Autodesk Fusion 360 part; units mm, degrees
sketch "Sketch1" plane through (0, 0, 0) normal (0, 0, 1) x (1, 0, 0)
  line L0 (-9, -12) -> (-9, 12)
  line L1 (9, 12) -> (9, -12)
  line L2 (9, -21) -> (-9, 21) construction
  line L3 (-9, -21) -> (9, 21) construction
  line L4 (9, -7.5) -> (-9, -7.5)
  line L5 (-9, -7.5) -> (-9, 7.5)
  line L6 (-9, 7.5) -> (9, 7.5)
  line L7 (9, 7.5) -> (9, -7.5)
  line L8 (9, -7.5) -> (-9, 7.5) construction
  line L9 (-9, -7.5) -> (9, 7.5) construction
  circle A0 centre (0, 0) radius 2.75
  arc A1 (0, 21) -> (-9, 12) centre (0, 12) ccw
  arc A2 (9, 12) -> (0, 21) centre (0, 12) ccw
  arc A3 (0, -21) -> (9, -12) centre (0, -12) ccw
  arc A4 (-9, -12) -> (0, -21) centre (0, -12) ccw
  line L10 (0, -21.9731) -> (0, 33.0269) construction
  line L11 (2.0496, 8.45) -> (4.0992, 12)
  line L12 (4.0992, 12) -> (2.0496, 15.55)
  line L13 (2.0496, 15.55) -> (-2.0496, 15.55)
  line L14 (-2.0496, 15.55) -> (-4.0992, 12)
  line L15 (-4.0992, 12) -> (-2.0496, 8.45)
  line L16 (-2.0496, 8.45) -> (2.0496, 8.45)
  line L17 (2.0496, -15.55) -> (4.0992, -12)
  line L18 (4.0992, -12) -> (2.0496, -8.45)
  line L19 (2.0496, -8.45) -> (-2.0496, -8.45)
  line L20 (-2.0496, -8.45) -> (-4.0992, -12)
  line L21 (-4.0992, -12) -> (-2.0496, -15.55)
  line L22 (-2.0496, -15.55) -> (2.0496, -15.55)
  circle A5 centre (0, 12) radius 2
  circle A6 centre (0, -12) radius 2
  line L23 (-9, 0) -> (0, 0) construction
  line L24 (-3.75, 3.5) -> (-7.25, 3.5)
  line L25 (-7.25, 3.5) -> (-7.25, -3.5)
  line L26 (-7.25, -3.5) -> (-3.75, -3.5)
  line L27 (-3.75, -3.5) -> (-3.75, 3.5)
  line L28 (-3.75, 3.5) -> (-7.25, -3.5) construction
  line L29 (-7.25, 3.5) -> (-3.75, -3.5) construction
  point P0 (0, 12)
  point P1 (0, -12)
  point P2 (-5.5, 0)
  dimension "d14" = 18
  dimension "d15" = 42
  dimension "d16" = 18
  dimension "d17" = 15
  dimension "d18" = 5.5
  dimension "d19" = 9
  dimension "d20" = 12
  dimension "d21" = 12
  dimension "d22" = 3.55
  dimension "d23" = 3.55
  dimension "d24" = 4
  dimension "d25" = 4
  dimension "d26" = 3.5
  dimension "d27" = 7
  dimension "d28" = 3.5
extrude "Extrude1" add sketch "Sketch1" against normal blind 5 contours L0 L1 L4 A3 A4 | L0 L1 L4 L5 L6 L7 | L0 L1 L6 A1 A2 | L11 L12 L13 L14 L15 L16 | L17 L18 L19 L20 L21 L22 | L24 L25 L26 L27
extrude "Extrude2" add sketch "Sketch1" along normal blind 10 contours L0 L1 L4 L5 L6 L7 | L24 L25 L26 L27
extrude "Extrude3" cut sketch "Sketch1" against normal blind 3.5 draft -5 contours L11 L12 L13 L14 L15 L16 | L17 L18 L19 L20 L21 L22 | A5 | A6
extrude "Extrude4" cut sketch "Sketch1" against normal blind 5 from surface at 10 contours L24 L25 L26 L27
sketch "Sketch2" plane through (-3.75, 0, 0) normal (-1, 0, 0) x (0, 0, 1)
  line L0 (10, -3.5) -> (10, 3.5)
  line L1 (10, 3.5) -> (5, 3.5)
  line L2 (5, 3.5) -> (5, -3.5)
  line L3 (5, -3.5) -> (10, -3.5)
  line L4 (9.0415, 0) -> (7.0207, 3.5)
  line L5 (7.0207, 3.5) -> (2.9793, 3.5)
  line L6 (2.9793, 3.5) -> (0.9585, 0)
  line L7 (0.9585, 0) -> (2.9793, -3.5)
  line L8 (2.9793, -3.5) -> (7.0207, -3.5)
  line L9 (7.0207, -3.5) -> (9.0415, 0)
  circle A0 centre (5, 0) radius 2.1
  point P0 (5, 0)
  dimension "d38" = 3.5
  dimension "d41" = 4.2
extrude "Extrude5" cut sketch "Sketch2" along normal up to surface (3.5 mm away) contours L1 L2 L3 L4 L5 L8 L9 A0 | L2 L5 L6 L7 L8 A0 | L2 A0 | L2 A0
extrude "Extrude6" cut sketch "Sketch2" against normal blind 9 from surface at 5.25 contours L2 A0 | L2 A0
chamfer "Chamfer1" distance 0.5 angle 45 19 edges at (-2.5639, 0.9944, 10) (-5.5, 3.5, 10) (-5.5, -3.5, 10) (-7.25, 0, 10) (-9, 0.7594, 3.0421) (-9, 9.75, 0) (0, 21, 0) (9, 9.75, 0) (0, -21, 0) (9, -9.75, 0) (-9, -9.75, 0) (0, 7.5, 10) (9, 0, 10) (0, -7.5, 10) (-9, 0, 10) (-9, 0, -5) (0, 21, -5) (9, 0, -5) (0, -21, -5)
chamfer "Chamfer1" distance 0.5 angle 45 1 edges at (-3.75, 0, 10)
Work out the finished part from the listing and answer in its coordinate system (mm). A direction names the side the tool comes from. Give positions to 0.01 mm unless a question says otherwise; leave off trailing zeros. Order: outer loops, then holes, each group sorted by start corner. A loop starts at its lowest first (then second) coordinate and runs counter-clockwise, first axis right, second up. Notation, with made-up numbers: (82, -14.75) -> (90, -14.75) arc R11 cw to (90, 4.25) -> close; hole circle Ø3 at (34.5, 85.5). An arc over 180 degrees is marked (long way). Answer as a JSON object with one key per item and string values. Group by question number.
1. A tool of negligible diameter and unlimited length cuts with its end or side. For faces 5 (the flat face through (0, 17, 0)), 6 (the cylindrical face through (-7.884, 0.631, 7.003)), 7 (the flat face through (0, -8.6, -1.7)), from which of +Z, -Z, +X, -X, +Y, -Y can it reach the whole face along a straight path? Write none if from no direction.
2. Flat-ended cylindrical pins translate along their axes: pin 1 Ø5 at (y, z) = (0, 5) entering from -X; pin 2 Ø1.9 at (x, y) = (1, 10.5) entering from +Z; pin 3 Ø1 at (x, z) = (-5.5, 6) entering from +Y; pin 4 Ø3.5 at (x, y) = (0, -12) entering from +Z. Find the tip coordinate at first contact, or state that the pin passes through.
3. The mould has two halves that part along X. Classify faces 1 (the flat face through (-6, -3.5, 6)), 2 (the flat face through (0, -7.5, 4)), 3 (the conical face through (-0.19, -20.64, -4.86)), 4 (the cylindrical face through (0, -10, -2)): released by +X, released by -X, zero draft, split by the parting line, or undercut.
4. Section C-C on x = 0 is taken. Count the separate pieces of the cut face and the enclosed holes in it, plus the area to 3 significant figures.
5. Consider line 1 along Y through (x, z) = (-8, 5); line 2 along Z through (x, y) = (-8.05, 0); line 3 along Y through (x, z) = (-4.5, 4.5). Determine where each line is inside the solid, lowest interval first. Write a range as [from, to].
6. Section B-B on z = 5 is taken. Determine the outline of the cut face in (x, y), plus the area to 3 significant figures.
7. Section A-A on y = -8 is taken. Determine the outline of the cut face in (x, z).
Result sheet:
{
 "1": {"face 5": "+Z, +X, -X, +Y", "face 6": "-X", "face 7": "+Z"},
 "2": {"pin 1": "stops at x = -8.9", "pin 2": "stops at z = 0", "pin 3": "stops at y = 7.5", "pin 4": "passes through"},
 "3": {"face 1": "undercut", "face 2": "zero draft", "face 3": "split by the parting line", "face 4": "undercut"},
 "4": {"separate pieces": "4", "enclosed holes": "0", "area": "219 mm^2"},
 "5": {"line 1": "y = [-7.5, -2.1], [2.1, 7.5]", "line 2": "z = [-5, 2.9], [7.1, 10]", "line 3": "y = [-7.5, -3.5], [3.5, 7.5]"},
 "6": {"outline": "(-9, -7.5) -> (9, -7.5) -> (9, 7.5) -> (-9, 7.5) -> (-9, 2.6) -> (-8.5, 2.1) -> (-7.25, 2.1) -> (-7.25, 3.5) -> (-3.75, 3.5) -> (-3.75, 2.1) -> (-1.78, 2.1) arc R2.75 cw (long way) to (-1.78, -2.1) -> (-3.75, -2.1) -> (-3.75, -3.5) -> (-7.25, -3.5) -> (-7.25, -2.1) -> (-8.5, -2.1) -> (-9, -2.6) -> close", "area": "209 mm^2"},
 "7": {"outline": "(-9, -4.5) -> (-8.5, -5) -> (8.5, -5) -> (9, -4.5) -> (9, -0.5) -> (8.5, 0) -> (-8.5, 0) -> (-9, -0.5) -> close"}
}
